Check sheet for the modelled part. Datum: model origin and axes. Units: mm. Face numbers are marked on the shaded views. A direction names the side the tool comes from. Give positions to 0.01 mm unless a question says otherwise; leave off trailing zeros. Loops run counter-clockwise (first coordinate to the right, second up) from the corner with the lowest first, then second, coordinate; pieces in that order, holes last. Notation, with made-up numbers: (-6, 85.25) - (5, 85.25) arc R13 ccw to (5, 91.25) - close; hole circle Ø7 at (42.25, 80). An arc over 180 degrees is marked (long way). Answer in a Markdown table with one row per item. Add a question column.
(1) Draft check along Z on the marked faces 5, 6 and 7. Enter one of: released by +Z, released by -Z, zero draft, split by the parting line, or undercut.
(2) Sectioned sample at B-B on z = 0. Enter the section's corners in (x, y), then the cut area to 3 significant figures.
(3) Sectioned sample at C-C on y = 6.5. Enter the section's corners in (x, z) (3 decimals), then the cut area to 3 significant figures.
(4) Thickness scan on L1, parallel to X at y = 4.5, z = 0.25; L2, parallel to Y at x = -8.75, z = 9.25; L3, parallel to Z at x = 0, y = 6.5 (3 decimals). Record the ranges inside material, lowest first.
(5) Go/stop test with flat-tipped pins: P1, Ø1.8, axis at y = 7, z = 1.5, coming from the +X side; P2, Ø5, axis at x = 11, y = 4, coming from the +Z side; P3, Ø0.6, axis at x = 12.5, y = 1, coming from the +Z side. Record where each tip stops, or that it passes through.
(6) Sectioned sample at A-A on x = 0. Enter the section's corners in (y, z) (3 decimals), then the cut area to 3 significant figures.
(7) Sectioned sample at D-D on x = 6. Enter the section's corners in (y, z).
(8) Set-up check for the marked faces 1, 2, 3 and 4: record each of +Z, -Z, +X, -X, +Y, -Y from which the full face is reachable in a straight line by a thin tool's end or side.
from build123d import *

# Parameters (mm, degrees)
EXTRUS_O1_DEPTH = 8.3
EXTRUS_O2_DEPTH = 7.3
ESCALA3_SCALE   = 1.1
ESBO_O3_R       = 15
EXTRUS_O3_DEPTH = 2
EXTRUS_O4_DEPTH = 23.379385604
ESBO_O5_W       = 4.083358115
ESBO_O5_H       = 1.749439388
ESBO_O5_W_2     = 1.749439388
ESBO_O5_H_2     = 4.083358115
EXTRUS_O5_DEPTH = 2


with BuildPart() as part:
    # Esboço1 → Extrusão1 (new body)
    with BuildSketch(Plane(origin=(0, 0, 0), x_dir=(1, 0, 0), z_dir=(0, 1, 0))):
        with BuildLine():
            Line((3.9, 0), (0, 0))
            Line((0, 0), (-3.9, 0))
            Line((-3.9, 0), (-3.9, -2.711549373))
            ThreePointArc((-3.9, -2.711549373), (0, -4.75), (3.9, -2.711549373))
            Line((3.9, -2.711549373), (3.9, 0))
        make_face()
        with BuildLine():
            Line((-3.9, 0), (0, 0))
            Line((0, 0), (3.9, 0))
            Line((3.9, 0), (3.9, 2.711549373))
            ThreePointArc((3.9, 2.711549373), (0, 4.75), (-3.9, 2.711549373))
            Line((-3.9, 2.711549373), (-3.9, 0))
        make_face()
        with BuildLine():
            Line((-3.9, 0), (0, 0))
            Line((0, 0), (3.9, 0))
            Line((3.9, 0), (3.9, 2.711549373))
            ThreePointArc((3.9, 2.711549373), (0, 4.75), (-3.9, 2.711549373))
            Line((-3.9, 2.711549373), (-3.9, 0))
        make_face()
    extrude(amount=EXTRUS_O1_DEPTH)

    # Esboço2 → Extrusão2 (cut)
    with BuildSketch(Plane(origin=(0, 8.3, 0), x_dir=(1, 0, 0), z_dir=(0, 1, 0))):
        with BuildLine():
            Line((-1.9, 0), (0, 0))
            Line((0, 0), (1.9, 0))
            Line((1.9, 0), (1.9, 1.988089535))
            ThreePointArc((1.9, 1.988089535), (0, 2.75), (-1.9, 1.988089535))
            Line((-1.9, 1.988089535), (-1.9, 0))
        make_face()
        with BuildLine():
            Line((1.9, 0), (0, 0))
            Line((0, 0), (-1.9, 0))
            Line((-1.9, 0), (-1.9, -1.988089535))
            ThreePointArc((-1.9, -1.988089535), (0, -2.75), (1.9, -1.988089535))
            Line((1.9, -1.988089535), (1.9, 0))
        make_face()
    extrude(amount=-EXTRUS_O2_DEPTH, mode=Mode.SUBTRACT)


with BuildPart() as part_1:
    # Escala3: scaled about (0, 0, 0)
    add(part.part.scale(ESCALA3_SCALE))

    # Esboço3 → Extrusão3 (add)
    with BuildSketch(Plane(origin=(0, 0, 0), x_dir=(1, 0, 0), z_dir=(0, 1, 0))):
        with Locations(Location((0, 0, 0), (0, 0, 270))):
            Circle(ESBO_O3_R)
    extrude(amount=EXTRUS_O3_DEPTH)

    # Esboço4 → Extrusão4 (cut, through all)
    with BuildSketch(Plane(origin=(0, 2, 0), x_dir=(1, 0, 0), z_dir=(0, 1, 0))):
        with BuildLine():
            Line((2.09, -2.186898489), (2.09, 2.186898489))
            ThreePointArc((2.09, 2.186898489), (0, 3.025), (-2.09, 2.186898489))
            Line((-2.09, 2.186898489), (-2.09, -2.186898489))
            ThreePointArc((-2.09, -2.186898489), (0, -3.025), (2.09, -2.186898489))
        make_face()
    extrude(amount=-EXTRUS_O4_DEPTH, mode=Mode.SUBTRACT)

    # Esboço5 → Extrusão5 (cut)
    with BuildSketch(Plane.XZ):
        Polygon((-2.14724761, -9.439201012), (-3.409074662, -13.322705355), (-5.072890392, -12.782098853), (-3.81106334, -8.89859451), align=None)
        Polygon((-4.959027358, -8.313677628), (-7.359165037, -11.617183737), (-8.774491233, -10.588889065), (-6.374353553, -7.285382956), align=None)
        Polygon((-7.285382956, -6.374353553), (-10.588889065, -8.774491233), (-11.617183737, -7.359165037), (-8.313677628, -4.959027358), align=None)
        Polygon((3.81106334, -8.89859451), (5.072890392, -12.782098853), (3.409074662, -13.322705355), (2.14724761, -9.439201012), align=None)
        Polygon((6.374353553, -7.285382956), (8.774491233, -10.588889065), (7.359165037, -11.617183737), (4.959027358, -8.313677628), align=None)
        Polygon((8.313677628, -4.959027358), (11.617183737, -7.359165037), (10.588889065, -8.774491233), (7.285382956, -6.374353553), align=None)
        Polygon((9.439201012, -2.14724761), (13.322705355, -3.409074662), (12.782098853, -5.072890392), (8.89859451, -3.81106334), align=None)
        with Locations((11.682428691, 0)):
            Rectangle(ESBO_O5_W, ESBO_O5_H)
        Polygon((8.89859451, 3.81106334), (12.782098853, 5.072890392), (13.322705355, 3.409074662), (9.439201012, 2.14724761), align=None)
        Polygon((4.959027358, 8.313677628), (7.359165037, 11.617183737), (8.774491233, 10.588889065), (6.374353553, 7.285382956), align=None)
        with Locations((0, 11.682428691)):
            Rectangle(ESBO_O5_W_2, ESBO_O5_H_2)
        Polygon((-3.81106334, 8.89859451), (-5.072890392, 12.782098853), (-3.409074662, 13.322705355), (-2.14724761, 9.439201012), align=None)
        with Locations((-11.682428691, 0)):
            Rectangle(ESBO_O5_W, ESBO_O5_H)
        Polygon((-8.89859451, -3.81106334), (-12.782098853, -5.072890392), (-13.322705355, -3.409074662), (-9.439201012, -2.14724761), align=None)
        with Locations((0, -11.682428691)):
            Rectangle(ESBO_O5_W_2, ESBO_O5_H_2)
        Polygon((8.313677628, 4.959027358), (7.285382956, 6.374353553), (10.588889065, 8.774491233), (11.617183737, 7.359165037), align=None)
        Polygon((2.14724761, 9.439201012), (3.409074662, 13.322705355), (5.072890392, 12.782098853), (3.81106334, 8.89859451), align=None)
        Polygon((-7.359165037, 11.617183737), (-8.774491233, 10.588889065), (-6.374353553, 7.285382956), (-4.959027358, 8.313677628), align=None)
        Polygon((-10.588889065, 8.774491233), (-11.617183737, 7.359165037), (-8.313677628, 4.959027358), (-7.285382956, 6.374353553), align=None)
        Polygon((-12.782098853, 5.072890392), (-13.322705355, 3.409074662), (-9.439201012, 2.14724761), (-8.89859451, 3.81106334), align=None)
    extrude(amount=-EXTRUS_O5_DEPTH, mode=Mode.SUBTRACT)


solid = part_1.part
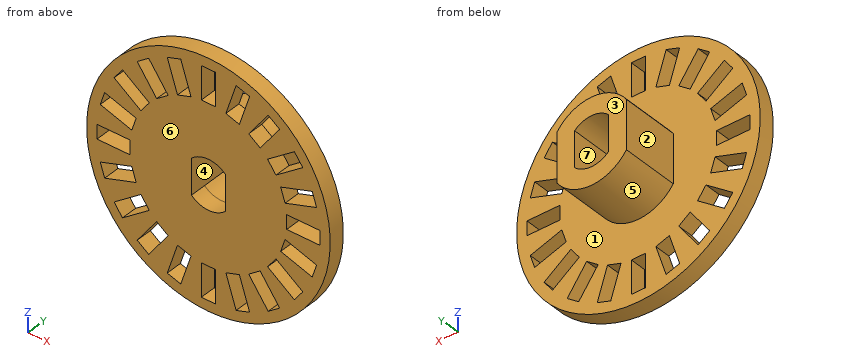
Reply:
| question | item | result |
|---|---|---|
| 1 | face 5 | released by -Z |
| 1 | face 6 | zero draft |
| 1 | face 7 | undercut |
| 2 | outline | (-15, 0) - (-13.72, 0) - (-13.72, 2) - (-15, 2) - close; (-9.64, 0) - (-2.09, 0) - (-2.09, 9.13) - (-4.29, 9.13) - (-4.29, 2) - (-9.64, 2) - close; (2.09, 0) - (9.64, 0) - (9.64, 2) - (4.29, 2) - (4.29, 9.13) - (2.09, 9.13) - close; (13.72, 0) - (15, 0) - (15, 2) - (13.72, 2) - close |
| 2 | area | 66.7 mm^2 |
| 3 | outline | (-4.29, -2.983) arc R5.225 ccw to (4.29, -2.983) - (4.29, 2.983) arc R5.225 ccw to (-4.29, 2.983) - close; hole (-2.09, -2.187) arc R3.025 ccw to (2.09, -2.187) - (2.09, 2.187) arc R3.025 ccw to (-2.09, 2.187) - close |
| 3 | area | 55.1 mm^2 |
| 4 | L1 | -4.29 to -2.09, 2.09 to 4.29 |
| 4 | L2 | 0 to 2 |
| 4 | L3 | -5.225 to -3.025, 3.025 to 5.225 |
| 5 | P1 | x = 4.29 |
| 5 | P2 | z = 11.61 |
| 5 | P3 | z = 8.73 |
| 6 | outline | (0, -15) - (2, -15) - (2, -13.724) - (0, -13.724) - close; (0, -9.641) - (2, -9.641) - (2, -5.225) - (9.13, -5.225) - (9.13, -3.025) - (0, -3.025) - close; (0, 3.025) - (9.13, 3.025) - (9.13, 5.225) - (2, 5.225) - (2, 9.641) - (0, 9.641) - close; (0, 13.724) - (2, 13.724) - (2, 15) - (0, 15) - close |
| 6 | area | 62.9 mm^2 |
| 7 | outline | (0, -13.75) - (2, -13.75) - (2, -9.75) - (0, -9.75) - close; (0, -7.56) - (2, -7.56) - (2, 7.56) - (0, 7.56) - close; (0, 9.75) - (2, 9.75) - (2, 13.75) - (0, 13.75) - close |
| 8 | face 1 | +Y |
| 8 | face 2 | +Z, -Z, -X, +Y |
| 8 | face 3 | +Z, -Z, +X, -X, +Y |
| 8 | face 4 | +Y, -Y |
